from build123d import *

# Parameters (mm, degrees)
SKETCH_1_W             = 28
SKETCH_1_H             = 30
SKETCH_1_R             = 9
EXTRUDE_1_DEPTH        = 8
SKETCH_2_R             = 11
SKETCH_2_R_2           = 9
EXTRUDE_2_DEPTH        = 2.5
SKETCH_3_R             = 10
SKETCH_3_R_2           = 9
EXTRUDE_3_DEPTH        = 4
HOLE_WIZARD_M3_1_D     = 2.5
HOLE_WIZARD_M3_1_DEPTH = 10
HOLE_WIZARD_M3_1_TIP   = 0.751075774
HOLE_WIZARD_M3_2_D     = 2.5
HOLE_WIZARD_M3_2_DEPTH = 10
HOLE_WIZARD_M3_2_TIP   = 0.751075774


with BuildPart() as part:
    # 草图1 → 凸台-拉伸1 (new body)
    with BuildSketch(Plane.XY):
        Rectangle(SKETCH_1_W, SKETCH_1_H)
        Circle(SKETCH_1_R, mode=Mode.SUBTRACT)
    extrude(amount=EXTRUDE_1_DEPTH)

    # 草图2 → 凸台-拉伸2 (add)
    with BuildSketch(Plane.XY.offset(8)):
        with Locations(Location((0, 0, 0), (0, 0, 180))):
            Circle(SKETCH_2_R)
        Circle(SKETCH_2_R_2, mode=Mode.SUBTRACT)
    extrude(amount=EXTRUDE_2_DEPTH)

    # 草图3 → 凸台-拉伸3 (add)
    with BuildSketch(Plane.XY.offset(10.5)):
        Circle(SKETCH_3_R)
        Circle(SKETCH_3_R_2, mode=Mode.SUBTRACT)
    extrude(amount=EXTRUDE_3_DEPTH)

    # M3 螺纹孔1
    with Locations(Plane(origin=(0, 15, 0), x_dir=(1, 0, 0), z_dir=(0, 1, 0))):
        with Locations((-10, -4), (10, -4)):
            Hole(HOLE_WIZARD_M3_1_D / 2, depth=HOLE_WIZARD_M3_1_DEPTH)
            with Locations((0, 0, -(HOLE_WIZARD_M3_1_DEPTH + HOLE_WIZARD_M3_1_TIP / 2))):  # 118° drill point
                Cone(0, HOLE_WIZARD_M3_1_D / 2, HOLE_WIZARD_M3_1_TIP, mode=Mode.SUBTRACT)

    # M3 螺纹孔2
    with Locations(Plane(origin=(0, -15, 0), x_dir=(-1, 0, 0), z_dir=(0, -1, 0))):
        with Locations((-10, -4), (10, -4)):
            Hole(HOLE_WIZARD_M3_2_D / 2, depth=HOLE_WIZARD_M3_2_DEPTH)
            with Locations((0, 0, -(HOLE_WIZARD_M3_2_DEPTH + HOLE_WIZARD_M3_2_TIP / 2))):  # 118° drill point
                Cone(0, HOLE_WIZARD_M3_2_D / 2, HOLE_WIZARD_M3_2_TIP, mode=Mode.SUBTRACT)


solid = part.part
For this review, take the finished solid that the model builds, in its own axes (mm). A direction names the side the tool comes from. Give positions to 0.01 mm unless a question says otherwise; leave off trailing zeros. Order: outer loops, then holes, each group sorted by start corner. A loop starts at its lowest first (then second) coordinate and runs counter-clockwise, first axis right, second up. Notation, with made-up numbers: (68, 89.5) - (127, 89.5) arc R34 cw to (127, 121.5) - close; hole circle Ø2 at (-21, -27). An arc over 180 degrees is marked (long way). Answer as a JSON object with one key per item and string values. Group by question number.
Item 1: Take a section at C-C on y = 0. Give the boundary of the cut face in (x, z), and give its area (3 significant figures).
Item 2: Take a section at B-B on y = -8. Give the boundary of the cut face in (x, z), and give its area (3 significant figures).
Item 3: Draft analysis for pull direction Z (two halves, no side actions). For faces 4 (the conical face through (10.028, -4.379, 3.785)), 5 (the flat face through (-2, 10, 10.5)), 6 (the cylindrical face through (-1.172, 8.923, 7.148)), state which applies: pulls with the +Z half, pulls with the -Z half, needs draft (parallel to the pull), parting line crosses it, or undercut.
Item 4: Machinability: for faces 1 (the cylindrical face through (-10.99, -9.93, 4.76)), 2 (the cylindrical face through (10.99, 9.93, 4.76)), 3 (the cylindrical face through (2.38, 10.74, 9.23)), which of the approach directions +Z, -Z, +X, -X, +Y, -Y give a long, thin tool a straight path to every point of the face, cutting with its end or side? Answer none if there is none.
Item 5: Take a section at A-A on x = 0. Give the boundary of the cut face in (y, z).
Item 6: Take a section at D-D on z = 2. Give the boundary of the cut face in (x, y), and give its area (3 significant figures).
Item 7: Wall thickness on line 1 along X through (y, z) = (11.75, 4); line 2 along Z through (x, y) = (-10, -10.5); line 3 along X through (y, z) = (-8, 4): over which ranges is each line inside the solid? List them lowest first.
Item 8: Clearance check with flat-ended pins moving along their axes: pin 1 Ø2 at (x, z) = (10, 4) entering from -Y; pin 2 Ø2 at (x, z) = (-10, 4) entering from +Y. State where each tip first meets the part, or that it passes through.
Reported:
{
 "1": {"outline": "(-14, 0) - (-9, 0) - (-9, 14.5) - (-10, 14.5) - (-10, 10.5) - (-11, 10.5) - (-11, 8) - (-14, 8) - close; (9, 0) - (14, 0) - (14, 8) - (11, 8) - (11, 10.5) - (10, 10.5) - (10, 14.5) - (9, 14.5) - close", "area": "98.0 mm^2"},
 "2": {"outline": "(-14, 0) - (-4.12, 0) - (-4.12, 14.5) - (-6, 14.5) - (-6, 10.5) - (-7.55, 10.5) - (-7.55, 8) - (-14, 8) - close; (4.12, 0) - (14, 0) - (14, 8) - (7.55, 8) - (7.55, 10.5) - (6, 10.5) - (6, 14.5) - (4.12, 14.5) - close; hole circle Ø2.5 at (-10, 4); hole circle Ø2.5 at (10, 4)", "area": "180 mm^2"},
 "3": {"face 4": "undercut", "face 5": "pulls with the +Z half", "face 6": "needs draft"},
 "4": {"face 1": "-Y", "face 2": "+Y", "face 3": "+Z"},
 "5": {"outline": "(-15, 0) - (-9, 0) - (-9, 14.5) - (-10, 14.5) - (-10, 10.5) - (-11, 10.5) - (-11, 8) - (-15, 8) - close; (9, 0) - (15, 0) - (15, 8) - (11, 8) - (11, 10.5) - (10, 10.5) - (10, 14.5) - (9, 14.5) - close"},
 "6": {"outline": "(-14, -15) - (14, -15) - (14, 15) - (-14, 15) - close; hole circle Ø18 at (0, 0)", "area": "586 mm^2"},
 "7": {"line 1": "-14 to -11.25, -8.75 to 8.75, 11.25 to 14", "line 2": "0 to 2.75, 5.25 to 8", "line 3": "-14 to -11.25, -8.75 to -4.12, 4.12 to 8.75, 11.25 to 14"},
 "8": {"pin 1": "y = -4.85", "pin 2": "y = 4.85"}
}
